For this review, take the finished solid that the model builds, in its own axes (mm). Round coordinates to 2 decimals unless told otherwise and drop trailing zeros. Order: outer loops, then holes, each group sorted by start corner. A loop starts at its lowest first (then second) coordinate and runs counter-clockwise, first axis right, second up. Notation, with made-up numbers: (11, 40.5) -> (23, 40.5) arc R29 ccw to (23, 74.5) -> close; hole circle Ø8 at (52.5, 55.5). An arc over 180 degrees is marked (long way). Answer in a Markdown table with one row per item.
```python
from build123d import *

# Parameters (mm, degrees)
F0_R     = 14.2875
F0_R_2   = 11
F1_DEPTH = 7
F3_DEPTH = 7
F4_COUNT = 3


with BuildPart() as f1:
    # F0 (on Top) → F1 (new body)
    with BuildSketch(Plane.XY):
        Circle(F0_R)
        Circle(F0_R_2, mode=Mode.SUBTRACT)
    extrude(amount=F1_DEPTH)

    # F2 (on face) → F3 (join)
    with BuildSketch(Plane.XY.offset(7)):
        with BuildLine():
            ThreePointArc((14.255938, 0.949145), (25.689929, 10.989739), (36.214913, 0))
            ThreePointArc((36.214913, 0), (25.689929, -10.989739), (14.255938, -0.949145))
            ThreePointArc((14.255938, -0.949145), (13.989619, -2.90228), (13.457006, -4.80017))
            ThreePointArc((13.457006, -4.80017), (27.660786, -12.462251), (37.914913, 0))
            ThreePointArc((37.914913, 0), (27.660786, 12.462251), (13.457006, 4.80017))
            ThreePointArc((13.457006, 4.80017), (13.989619, 2.90228), (14.255938, 0.949145))
        make_face()
    extrude(amount=-F3_DEPTH)

    # F4: F1 ×3 about axis
    f4_axis = Axis((0, 0, 7), (0, 0, 1))


with BuildPart() as f1_1:
    add(f1.part)
    for i in range(1, F4_COUNT):
        add(f1.part.rotate(f4_axis, i * 360 / F4_COUNT))


solid = f1_1.part
```
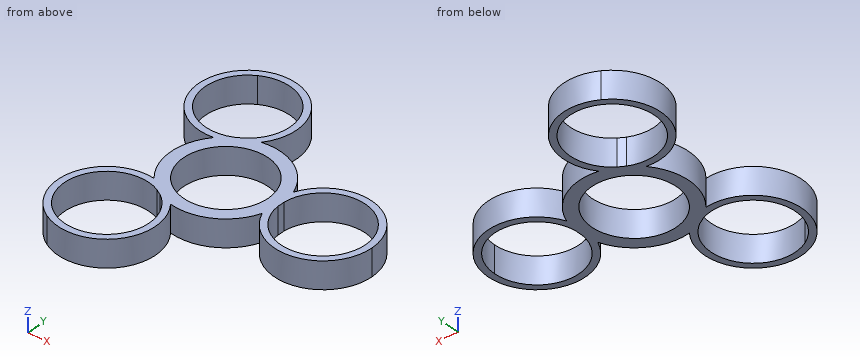
Q1. Take a section at A-A, the plane z = 5.5. Write out the cut boundary in (x, y) (1 decimal), then the cut area to 3 significant figures.
Answer key:
| item | result |
|---|---|
| outline | (-10.9, -9.3) arc R12.7 ccw (long way) to (-2.6, -14.1) arc R14.3 ccw to (13.5, -4.8) arc R12.7 ccw (long way) to (13.5, 4.8) arc R14.3 ccw to (-2.6, 14.1) arc R12.7 ccw (long way) to (-10.9, 9.3) arc R14.3 ccw to start; hole circle Ø22 at (0, 0); hole (-7.9, -11.9) arc R11 ccw (long way) to (-6.3, -12.8) arc R14.3 cw to start; hole (-7.9, 11.9) arc R14.3 cw to (-6.3, 12.8) arc R11 ccw (long way) to start; hole (14.3, -0.9) arc R11 ccw (long way) to (14.3, 0.9) arc R14.3 cw to start |
| area | 607 mm^2 |
Q2. To check wall thickness, follow probe 1 along X at (y, z) = (0, 5); probe 2 along X at (y, z) = (-1.5, 3.25); probe 3 along Y at (x, z) = (-10, 4.25). State the ranges of each line that lie inside material, in increasing order.
Answer key:
| item | result |
|---|---|
| probe 1 | x = -14.29 to -11, 11 to 14.29, 36.21 to 37.91 |
| probe 2 | x = -14.21 to -10.9, 10.9 to 14.32, 36.11 to 37.83 |
| probe 3 | y = -34.27 to -32.52, -11.15 to -4.58, 4.58 to 11.15, 32.52 to 34.27 |
Q3. Clearance check with flat-ended pins moving along their axes: pin 1 Ø3 at (x, z) = (-15, 2.5) entering from +Y; pin 2 Ø17.5 at (x, y) = (0, 0) entering from +Z; pin 3 Ø2 at (x, z) = (17.5, 1) entering from -Y. State where each tip first meets the part, or that it passes through.
Answer key:
| item | result |
|---|---|
| pin 1 | stops at y = 34.51 |
| pin 2 | passes through |
| pin 3 | stops at y = -10.78 |
Q4. Take a section at B-B, the plane x = 27. Write out the cut boundary in (y, z), then the cut area to 3 significant figures.
Answer key:
| item | result |
|---|---|
| outline | (-12.57, 0) -> (-10.85, 0) -> (-10.85, 7) -> (-12.57, 7) -> close; (10.85, 0) -> (12.57, 0) -> (12.57, 7) -> (10.85, 7) -> close |
| area | 24.1 mm^2 |
Q5. Take a section at C-C, the plane y = 29. Write out the cut boundary in (x, z), then the cut area to 3 significant figures.
Answer key:
| item | result |
|---|---|
| outline | (-23.09, 0) -> (-20.96, 0) -> (-20.96, 7) -> (-23.09, 7) -> close; (-4.26, 0) -> (-2.12, 0) -> (-2.12, 7) -> (-4.26, 7) -> close |
| area | 29.9 mm^2 |
